Verification items for the finished model (mm, model axes). A direction names the side the tool comes from. Give positions to 0.01 mm unless a question says otherwise; leave off trailing zeros. Loops run counter-clockwise (first coordinate to the right, second up) from the corner with the lowest first, then second, coordinate; pieces in that order, holes last. Notation, with made-up numbers: (78, 46.25) - (131, 46.25) arc R10 cw to (131, 55.25) - close; hole circle Ø11 at (11.5, 21.25). An arc over 180 degrees is marked (long way). One line per item, written item: value. Start each with the question number.
1. Sectioned sample at C-C (z = 3.1). Count the separate pieces of the cut face and the enclosed holes in it, plus the area to 3 significant figures.
2. Access from +Z, -Z, +X, -X, +Y, -Y to the whole of each face (thin tool, end or side, straight path). Record for faces 1 (the flat face through (64.5, -118, 2)), 2 (the flat face through (75.5, -4, 2)), 3 (the flat face through (141.84, -109.73, 2.35)), 4 (the flat face through (-2, -45.503, 2)), 5 (the cylindrical face through (-4.95, -42, 2.35)).
3. Sectioned sample at A-A (x = 70). Record the cut outline in (y, z), plus the area to 3 significant figures.
4. Scan lines: L1, parallel to Y at x = 70, z = 1.05; L2, parallel to Y at x = 71, z = 3.35; L3, parallel to X at y = -32.5, z = 2. Record each from-to range of solid material in increasing order. Write a range as [from, to].
5. Sectioned sample at B-B (y = -92). Record the cut outline in (x, z).
6. Gauge pin test, flat ends, axial feed: pin 1 (4 mm diameter, centred on x = 0.26, y = -5.93, fed in from -Z); pin 2 (2.5 mm diameter, centred on x = 40, z = 3.5, fed in from +Y); pin 3 (1.5 mm diameter, centred on y = -49, z = 4, fed in from +X); pin 4 (2 mm diameter, centred on y = -117, z = 2, fed in from +X). Record the tip position at first contact, or that the pin passes through.
7. Mould release check, pull along X, two halves, no side actions. Record for faces 6 (the flat face through (103, -115.669, 2)), 7 (the flat face through (69, -60, 0)), 8 (the flat face through (0, -76, 2)): pulls with the +X half, pulls with the -X half, needs draft (parallel to the pull), parting line crosses it, or undercut.
from build123d import *

# Parameters (mm, degrees)
BOSS_EXTRUDE1_DEPTH  = 4.7625
M4_CLEARANCE_HOLE1_D = 4.5


with BuildPart() as part:
    # Sketch1 → Boss-Extrude1 (new body)
    with BuildSketch(Plane.XY):
        with BuildLine():
            Line((-3.626904156, -9.820077826), (0, -13.446981982))
            Line((0, -13.446981982), (0, -33.529852105))
            Line((0, -33.529852105), (0, -34.502807389))
            Line((0, -34.502807389), (-3.9097, -34.502807389))
            ThreePointArc((-3.9097, -34.502807389), (-9.4097, -40.002807389), (-3.9097, -45.502807389))
            Line((-3.9097, -45.502807389), (0, -45.502807389))
            Line((0, -45.502807389), (0, -46.902807389))
            Line((0, -46.902807389), (0, -51.502807389))
            Line((0, -51.502807389), (0, -107.890632795))
            Line((0, -107.890632795), (-3.626904156, -111.517536951))
            ThreePointArc((-3.626904156, -111.517536951), (-3.626904156, -119.295711544), (4.151270437, -119.295711544))
            Line((4.151270437, -119.295711544), (7.778174593, -115.668807389))
            Line((7.778174593, -115.668807389), (64.5, -115.668807389))
            Line((64.5, -115.668807389), (64.5, -119.578507389))
            ThreePointArc((64.5, -119.578507389), (70, -125.078507389), (75.5, -119.578507389))
            Line((75.5, -119.578507389), (75.5, -115.668807389))
            Line((75.5, -115.668807389), (132.221825407, -115.668807389))
            Line((132.221825407, -115.668807389), (135.848729563, -119.295711544))
            ThreePointArc((135.848729563, -119.295711544), (143.626904156, -119.295711544), (143.626904156, -111.517536951))
            Line((143.626904156, -111.517536951), (140, -107.890632795))
            Line((140, -107.890632795), (140, -66.168807389))
            Line((140, -66.168807389), (143.9097, -66.168807389))
            ThreePointArc((143.9097, -66.168807389), (149.4097, -60.668807389), (143.9097, -55.168807389))
            Line((143.9097, -55.168807389), (140, -55.168807389))
            Line((140, -55.168807389), (140, -13.446981982))
            Line((140, -13.446981982), (143.626904156, -9.820077826))
            ThreePointArc((143.626904156, -9.820077826), (143.626904156, -2.041903233), (135.848729563, -2.041903233))
            Line((135.848729563, -2.041903233), (132.221825407, -5.668807389))
            Line((132.221825407, -5.668807389), (75.5, -5.668807389))
            Line((75.5, -5.668807389), (75.5, -1.759107389))
            ThreePointArc((75.5, -1.759107389), (70, 3.740892611), (64.5, -1.759107389))
            Line((64.5, -1.759107389), (64.5, -5.668807389))
            Line((64.5, -5.668807389), (7.778174593, -5.668807389))
            Line((7.778174593, -5.668807389), (4.151270437, -2.041903233))
            ThreePointArc((4.151270437, -2.041903233), (-3.626904156, -2.041903233), (-3.626904156, -9.820077826))
        make_face()
    extrude(amount=BOSS_EXTRUDE1_DEPTH)

    # M4 Clearance Hole1 (through all)
    with Locations(Plane.XY.offset(4.7625)):
        with Locations((0.262183141, -5.930990529), (-3.9097, -40.002807389), (0.262183141, -115.406624248), (70, -119.578507389), (139.737816859, -115.406624248), (143.9097, -60.668807389), (139.737816859, -5.930990529), (70, -1.759107389)):
            Hole(M4_CLEARANCE_HOLE1_D / 2)


solid = part.part
Results are:
1. separate pieces: 1
1. enclosed holes: 8
1. area: 15,900 mm^2
2. face 1: +Z, -Z, -Y
2. face 2: +Z, -Z, +Y
2. face 3: +Z, -Z, +X
2. face 4: +Z, -Z, -X
2. face 5: +Z, -Z
3. outline: (-125.08, 0) - (-121.83, 0) - (-121.83, 4.76) - (-125.08, 4.76) - close; (-117.33, 0) - (-4.01, 0) - (-4.01, 4.76) - (-117.33, 4.76) - close; (0.49, 0) - (3.74, 0) - (3.74, 4.76) - (0.49, 4.76) - close
3. area: 571 mm^2
4. L1: y = [-125.08, -121.83], [-117.33, -4.01], [0.49, 3.74]
4. L2: y = [-124.99, -121.59], [-117.56, -3.77], [0.26, 3.65]
4. L3: x = [0, 140]
5. outline: (0, 0) - (140, 0) - (140, 4.76) - (0, 4.76) - close
6. pin 1: passes through
6. pin 2: stops at y = -5.67
6. pin 3: stops at x = 140
6. pin 4: stops at x = 145.21
7. face 6: undercut
7. face 7: needs draft
7. face 8: pulls with the -X half
